CAD build for the part. Positions are in the model's coordinates, mm. A direction names the side the tool comes from. Coordinates: 2 decimals unless noted, no trailing zeros. Loops run counter-clockwise (first coordinate to the right, second up) from the corner with the lowest first, then second, coordinate; pieces in that order, holes last.
1) Pin check, flat tips, straight feed: pin 1 Ø5 at (x, z) = (-43.5, -11.5) entering from -Y; pin 2 Ø13.5 at (x, z) = (-2.5, -5.5) entering from -Y. Stop position of each tip, or through.
2) Saw through at D-D, the plane z = 0. Write the cut outline in (x, y).
3) Saw through at B-B, the plane x = 0. Write the cut outline in (y, z), and give its area (3 significant figures).
4) Saw through at C-C, the plane y = -25. Write the cut outline in (x, z).
5) Which spindle directions (+Z, -Z, +X, -X, +Y, -Y) get a long thin tool onto all of the face, cutting with end or side? Do faces 1 (the cylindrical face through (-3, -15.9, -13.4)), 2 (the flat face through (-69.85, -16, 0)). Say none if no direction does.
6) Wall check: line 1 along X through (y, z) = (-23, -18); line 2 along Z through (x, y) = (54, -30); line 3 along X through (y, z) = (-16, -8). Give the ranges that are in metal, low to high.
7) Saw through at A-A, the plane z = -17.5. Write the cut outline in (x, y).
8) Two-plate mould, pull along Z, no slides. Class faces 3 (the flat face through (-1, -16, 31.75)), 4 (the flat face through (-1, 0, 0)), 5 (the flat face through (-14, -12.7, 5)), 6 (the flat face through (-57.261, -22, 0)): +Z half, -Z half, draft (parallel to the pull), parting line (faces both ways), or undercut.
```python
from build123d import *

# Parameters (mm, degrees)
F0_W     = 139.7
F0_H     = 63.5
F1_DEPTH = 31.75
F2_W     = 114.522352
F2_H     = 46.118464
F3_DEPTH = 12.7
F4_W     = 114.522352
F4_H     = 46.118464
F4_R     = 13.731838
F5_DEPTH = 6.35


with BuildPart() as f1:
    # F0 (on Front) → F1 (new body)
    with BuildSketch(Plane.XZ):
        Rectangle(F0_W, F0_H)
    extrude(amount=F1_DEPTH)

    # F2 (on face) → F3 (cut)
    with BuildSketch(Plane.XZ.offset(31.75)):
        Rectangle(F2_W, F2_H)
    extrude(amount=-F3_DEPTH, mode=Mode.SUBTRACT)

    # F4 (on face) → F5 (cut)
    with BuildSketch(Plane.XZ.offset(19.05)):
        Rectangle(F4_W, F4_H)
        Circle(F4_R, mode=Mode.SUBTRACT)
    extrude(amount=-F5_DEPTH, mode=Mode.SUBTRACT)


solid = f1.part
```
Data:
1. pin 1: stops at y = -12.7
1. pin 2: stops at y = -19.05
2. outline: (-69.85, -31.75) - (-57.26, -31.75) - (-57.26, -12.7) - (-13.73, -12.7) - (-13.73, -19.05) - (13.73, -19.05) - (13.73, -12.7) - (57.26, -12.7) - (57.26, -31.75) - (69.85, -31.75) - (69.85, 0) - (-69.85, 0) - close
3. outline: (-31.75, -31.75) - (0, -31.75) - (0, 31.75) - (-31.75, 31.75) - (-31.75, 23.06) - (-12.7, 23.06) - (-12.7, 13.73) - (-19.05, 13.73) - (-19.05, -13.73) - (-12.7, -13.73) - (-12.7, -23.06) - (-31.75, -23.06) - close
3. area: 1,310 mm2
4. outline: (-69.85, -31.75) - (69.85, -31.75) - (69.85, 31.75) - (-69.85, 31.75) - close; hole (-57.26, -23.06) - (57.26, -23.06) - (57.26, 23.06) - (-57.26, 23.06) - close
5. face 1: -Y
5. face 2: +Z, -Z, -X, +Y, -Y
6. line 1: x = -69.85 to -57.26, 57.26 to 69.85
6. line 2: z = -31.75 to -23.06, 23.06 to 31.75
6. line 3: x = -69.85 to -57.26, -11.16 to 11.16, 57.26 to 69.85
7. outline: (-69.85, -31.75) - (-57.26, -31.75) - (-57.26, -12.7) - (57.26, -12.7) - (57.26, -31.75) - (69.85, -31.75) - (69.85, 0) - (-69.85, 0) - close
8. face 3: +Z half
8. face 4: draft
8. face 5: undercut
8. face 6: undercut
